from build123d import *

# Parameters (mm, degrees)
F1_DEPTH = 63.5
F2_DEPTH = 7.9375
F3_DEPTH = 25.4
F0_W     = 10.3774026796
F0_H     = 19.05
F5_R     = 5.08


with BuildPart() as f1:
    # F0 (on Front) → F1 (new body, symmetric)
    with BuildSketch(Plane.XZ):
        Polygon((-47.625, -9.525), (47.625, -9.525), (47.625, 9.525), (28.575, 9.525), (-47.625, 9.525), align=None)
    extrude(amount=F1_DEPTH, both=True)

    # F0 (on Front) → F2 (join, symmetric)
    with BuildSketch(Plane.XZ):
        with BuildLine():
            add(Edge.make_bspline(
                [(-47.625, 9.525), (-41.1829413646, 48.2544610148), (-3.609227819, 62.5325655632), (41.275, 62.8309662256)],
                knots=[0, 0, 0, 0, 105.7723986336, 105.7723986336, 105.7723986336, 105.7723986336], degree=3))
            Line((-47.625, 9.525), (28.575, 9.525))
            Line((28.575, 9.525), (28.575, 27.0002))
            ThreePointArc((28.575, 27.0002), (31.9091488719, 41.8922700374), (41.275, 53.9409683632))
            Line((41.275, 53.9409683632), (41.275, 62.8309662256))
        make_face()
    extrude(amount=F2_DEPTH, both=True)

    # F0 (on Front) → F3 (join, symmetric)
    with BuildSketch(Plane.XZ):
        with BuildLine():
            ThreePointArc((63.5, 42.8752), (57.3434465811, 41.6327826497), (52.1505478123, 38.1))
            Line((52.1505478123, 38.1), (92.075, 38.1))
            Line((92.075, 38.1), (92.075, 42.8752))
            Line((92.075, 42.8752), (63.5, 42.8752))
        make_face()
        with BuildLine():
            Line((41.275, 66.675), (41.275, 62.8309662256))
            add(Edge.make_bspline(
                [(41.275, 62.8309662256), (48.5260198489, 62.8791726721), (55.9678310127, 62.5625339124), (63.5, 61.9252)],
                knots=[105.7723986336, 105.7723986336, 105.7723986336, 105.7723986336, 122.8598656398, 122.8598656398, 122.8598656398, 122.8598656398], degree=3))
            Line((63.5, 61.9252), (92.075, 61.9252))
            Line((92.075, 61.9252), (92.075, 66.675))
            Line((92.075, 66.675), (41.275, 66.675))
        make_face()
        with BuildLine():
            add(Edge.make_bspline(
                [(41.275, 62.8309662256), (48.5260198489, 62.8791726721), (55.9678310127, 62.5625339124), (63.5, 61.9252)],
                knots=[105.7723986336, 105.7723986336, 105.7723986336, 105.7723986336, 122.8598656398, 122.8598656398, 122.8598656398, 122.8598656398], degree=3))
            Line((41.275, 62.8309662256), (41.275, 53.9409683632))
            ThreePointArc((41.275, 53.9409683632), (51.6921786532, 59.8685887655), (63.5, 61.9252))
        make_face()
        with BuildLine():
            Line((41.275, 38.1), (52.1505478123, 38.1))
            ThreePointArc((52.1505478123, 38.1), (57.3434465811, 41.6327826497), (63.5, 42.8752))
            Line((63.5, 42.8752), (92.075, 42.8752))
            Line((92.075, 42.8752), (92.075, 61.9252))
            Line((92.075, 61.9252), (63.5, 61.9252))
            ThreePointArc((63.5, 61.9252), (51.6921786532, 59.8685887655), (41.275, 53.9409683632))
            Line((41.275, 53.9409683632), (41.275, 38.1))
        make_face()
    extrude(amount=F3_DEPTH, both=True)

    # F0 (on Front) → F4 (revolve)
    with BuildSketch(Plane.XZ):
        with Locations((97.2637013398, 52.4002)):
            Rectangle(F0_W, F0_H)
    revolve(axis=Axis((92.075, 0, 52.3875), (0, 0, 1)))

    # F5
    f5_edges = [f1.edges().sort_by_distance(p)[0] for p in [
        (-47.625, -63.5, 0),
        (47.625, -63.5, 0),
        (47.625, 63.5, 0),
        (-47.625, 63.5, 0),
    ]]
    fillet(f5_edges, radius=F5_R)


solid = f1.part
Geometry: final body of the model. Coordinates: model frame, mm. A direction names the side the tool comes from. Give positions to 0.01 mm unless a question says otherwise; leave off trailing zeros. Loops run counter-clockwise (first coordinate to the right, second up) from the corner with the lowest first, then second, coordinate; pieces in that order, holes last. Notation, with made-up numbers: (76, -35) -> (102, -35) arc R23 ccw to (102, -26) -> close; hole circle Ø9 at (21.25, 2). An arc over 180 degrees is marked (long way). Put each result on its own line as item: value.
1. Cut plane B-B (z = -2.5). Return the cut outline in (x, y) (3 decimals), plus the area to 3 significant figures.
Taken from the geometry:
outline: (-47.625, -58.42) arc R5.08 ccw to (-42.545, -63.5) -> (42.545, -63.5) arc R5.08 ccw to (47.625, -58.42) -> (47.625, 58.42) arc R5.08 ccw to (42.545, 63.5) -> (-42.545, 63.5) arc R5.08 ccw to (-47.625, 58.42) -> close
area: 12,100 mm2
2. Pin query (flat end, axial travel): P1, Ø14.5, axis at x = 76, z = 55, coming from the +Y side; P2, Ø9.5, axis at y = -11, z = -0.5, coming from the +X side (3 decimals); P3, Ø3, axis at x = 99, y = 0, coming from the +Z side; P4, Ø8.5, axis at y = 1.5, z = 49.5, coming from the +X side. Return the tip coordinate at first contact, or that it passes through.
Taken from the geometry:
P1: stops at y = 25.4
P2: stops at x = 47.625
P3: stops at z = 61.93
P4: stops at x = 102.45
3. Cut plane A-A (y = 13). Return the cut outline in (x, z) (3 decimals).
Taken from the geometry:
outline: (-47.625, -9.525) -> (47.625, -9.525) -> (47.625, 9.525) -> (-47.625, 9.525) -> close; (41.275, 38.1) -> (92.075, 38.1) -> (92.075, 66.675) -> (41.275, 66.675) -> close
4. Ray query, line 1 along Z through (x, y) = (41.5, -17.5) (3 decimals); line 2 along Y through (x, z) = (78, 55.5); line 3 along X through (y, z) = (-10.5, 2) (3 decimals). Return the intervals inside material, ascending. Write a range as [from, to].
Taken from the geometry:
line 1: z = [-9.525, 9.525], [38.1, 66.675]
line 2: y = [-25.4, 25.4]
line 3: x = [-47.625, 47.625]
5. Cut plane D-D (y = -55.5). Return the cut outline in (x, z) (3 decimals), plus the area to 3 significant figures.
Taken from the geometry:
outline: (-47.625, -9.525) -> (47.625, -9.525) -> (47.625, 9.525) -> (-47.625, 9.525) -> close
area: 1,810 mm2
6. Cut plane C-C (x = 54). Return the cut outline in (y, z) (3 decimals).
Taken from the geometry:
outline: (-25.4, 38.1) -> (25.4, 38.1) -> (25.4, 66.675) -> (-25.4, 66.675) -> close
7. Set-up query: faces 1 (the flat face through (96, 0, 61.925)), 2 (the flat face through (47.625, -1, 0)), 3 (the flat face through (-3, 7.938, 31)), 4 (the flat face through (41.275, 0, 53)), 5 (the flat face through (-3, -7.938, 31)). Return all of +Z, -Z, +X, -X, +Y, -Y with unobstructed straight access to the full face (end or side cutting, diameter ignored); none if empty.
Taken from the geometry:
face 1: +Z, +X, +Y, -Y
face 2: -Z, +X, +Y, -Y
face 3: +Z, -X, +Y
face 4: none
face 5: +Z, -X, -Y
8. Pull-direction query (Z, two-part tool) for faces 6 (the flat face through (67, 0, 66.675)), 7 (the cylindrical face through (-46.18, 61.97, -0.13)), 8 (the flat face through (28.575, 0, 18)); classes: released by +Z, released by -Z, zero draft, split by the parting line, or undercut.
Taken from the geometry:
face 6: released by +Z
face 7: zero draft
face 8: undercut
